The model under review builds one solid part; all positions refer to its coordinate system, in mm. A direction names the side the tool comes from. Round coordinates to 2 decimals unless told otherwise and drop trailing zeros. Write each loop counter-clockwise with the first axis right and the second up, starting at its lowest first coordinate (ties: lowest second). Pieces come first, ordered by that corner, then holes. Notation, with made-up numbers: M 80,59 L 117,59 A9 cw 117,68 Z; hole C -22,48.25 d6. An arc over 180 degrees is marked long. One line per item, written item: value. Start each with the question number.
1) Mouldability with a two-part tool opening along X and no side actions: class faces 1 (the face through (-128.15, 0, 37)), 2 (the face through (-142.35, -6.72, 22.98)), 3 (the face through (-146.05, 0, 61)) as +X half, -X half, draft (parallel to the pull), parting line (faces both ways), or undercut.
2) For P1, Ø13, axis at y = 0, z = 31.75, coming from the -X side; P2, Ø4, axis at x = -2, y = -10, coming from the +Z side; P3, Ø4, axis at x = 110.5, y = -12, coming from the -Z side, all flat-tipped, find the tip position at first contact; note any pin that passes through.
3) Take a section at D-D, the plane y = 0. State how many separate pieces and enclosed holes the cut face has, and give its area (3 significant figures).
4) Tool access review of faces 4 (the face through (-102, 0, 0)), 5 (the face through (-88, 0, 19.05)), 6 (the face through (-37.5, 0, -5)), 7 (the face through (101, 0, 0)), 8 (the face through (-133.42, 1.22, 35.61)): name each direction out of +Z, -Z, +X, -X, +Y, -Y from which nothing blocks a thin tool from reaching the whole face with its end or side.
5) Take a section at A-A, the plane x = -44.5. Write out the cut boundary in (y, z) (3 decimals), and give its area (3 significant figures).
6) Take a section at C-C, the plane z = 31.75. Write out the cut boundary in (x, y) (3 decimals), and give its area (3 significant figures).
7) Wall thickness on probe 1 along X at (y, z) = (11, 111.5); probe 2 along X at (y, z) = (-7, 38); probe 3 along X at (y, z) = (4, -11): over which ranges is each line inside the solid? List them lowest first.
8) Take a section at B-B, the plane z = 82. Write out the cut boundary in (x, y) (3 decimals).
from build123d import *

# Parameters (mm, degrees)
SKETCH1_R           = 8.05
SKETCH1_R_2         = 7
SKETCH1_R_3         = 1.25
BOSS_EXTRUDE1_DEPTH = 15.875
SKETCH2_R           = 11.05
CUT_EXTRUDE1_DEPTH  = 7.5
CUT_EXTRUDE3_START  = -7.5
SKETCH3_R           = 11.05
CUT_EXTRUDE3_DEPTH  = 7.5
SKETCH4_R           = 4.05
CUT_EXTRUDE4_DEPTH  = 10.4
SKETCH5_W           = 4
SKETCH5_H           = 27.75
CUT_EXTRUDE5_DEPTH  = 191.102710725


with BuildPart() as part:
    # Sketch1 → Boss-Extrude1 (new, symmetric)
    with BuildSketch(Plane(origin=(0, 0, 0), x_dir=(1, 0, 0), z_dir=(0, 1, 0))):
        with BuildLine():
            Line((-146.05, 0), (-56.5, 0))
            ThreePointArc((-56.5, 0), (-44.5, 12), (-32.5, 0))
            Line((-32.5, 0), (-15.05, 0))
            ThreePointArc((-15.05, 0), (0, 15.05), (15.05, 0))
            Line((15.05, 0), (32.5, 0))
            ThreePointArc((32.5, 0), (44.5, 12), (56.5, 0))
            Line((56.5, 0), (146.05, 0))
            Line((146.05, 0), (146.05, -120.65))
            Line((146.05, -120.65), (133.35, -120.65))
            Line((133.35, -120.65), (133.35, -44.45))
            Line((133.35, -44.45), (-57.15, -44.45))
            Line((-57.15, -44.45), (-57.15, -19.05))
            Line((-57.15, -19.05), (-120.65, -19.05))
            Line((-120.65, -19.05), (-120.65, -120.65))
            Line((-120.65, -120.65), (-146.05, -120.65))
            Line((-146.05, -120.65), (-146.05, 0))
        make_face()
        with Locations(Location((0, 0, 0), (0, 0, 270))):
            Circle(SKETCH1_R, mode=Mode.SUBTRACT)
        with Locations(Location((-44.5, 0, 0), (0, 0, 270))):
            Circle(SKETCH1_R_2, mode=Mode.SUBTRACT)
        with Locations(Location((44.5, 0, 0), (0, 0, 270))):
            Circle(SKETCH1_R_2, mode=Mode.SUBTRACT)
        with Locations(Location((0, 11.25, 0), (0, 0, 270))):
            Circle(SKETCH1_R_3, mode=Mode.SUBTRACT)
        with Locations(Location((9.742785793, -5.625, 0), (0, 0, 270))):
            Circle(SKETCH1_R_3, mode=Mode.SUBTRACT)
        with Locations(Location((-9.742785793, -5.625, 0), (0, 0, 270))):
            Circle(SKETCH1_R_3, mode=Mode.SUBTRACT)
    extrude(amount=BOSS_EXTRUDE1_DEPTH, both=True)

    # Sketch2 → Cut-Extrude1 (cut)
    with BuildSketch(Plane.ZY.offset(146.05)):
        with Locations((31.75, 0)):
            Circle(SKETCH2_R)
    extrude(amount=-CUT_EXTRUDE1_DEPTH, mode=Mode.SUBTRACT)

    # Sketch3 → Cut-Extrude3 (cut)
    with BuildSketch(Plane(origin=(-120.65, 0, 0), x_dir=(0, 0, -1), z_dir=(1, 0, 0)).offset(CUT_EXTRUDE3_START)):
        with Locations(Location((-31.75, 0, 0), (0, 0, 180))):
            Circle(SKETCH3_R)
    extrude(amount=CUT_EXTRUDE3_DEPTH, mode=Mode.SUBTRACT)

    # Sketch4 → Cut-Extrude4 (cut)
    with BuildSketch(Plane.ZY.offset(138.55)):
        with Locations((31.75, 0)):
            Circle(SKETCH4_R)
    extrude(amount=-CUT_EXTRUDE4_DEPTH, mode=Mode.SUBTRACT)

    # Sketch5 → Cut-Extrude5 (cut, through all)
    with BuildSketch(Plane(origin=(0, 0, 0), x_dir=(-1, 0, 0), z_dir=(0, 0, -1))):
        with Locations((-49.5, 0)):
            Rectangle(SKETCH5_W, SKETCH5_H)
        with Locations((-39.5, 0)):
            Rectangle(SKETCH5_W, SKETCH5_H)
        with Locations((49.5, 0)):
            Rectangle(SKETCH5_W, SKETCH5_H)
        with Locations((39.5, 0)):
            Rectangle(SKETCH5_W, SKETCH5_H)
    extrude(amount=CUT_EXTRUDE5_DEPTH, mode=Mode.SUBTRACT)


solid = part.part
Checked values:
1. face 1: undercut
1. face 2: draft
1. face 3: -X half
2. P1: stops at x = -138.55
2. P2: stops at z = 44.45
2. P3: stops at z = 0
3. separate pieces: 4
3. enclosed holes: 4
3. area: 14,000 mm2
4. face 4: -Z, -X, +Y, -Y
4. face 5: +Z, +Y, -Y
4. face 6: -Z
4. face 7: -Z, +X, +Y, -Y
4. face 8: -X
5. outline: M -15.875,-12 L 15.875,-12 L 15.875,-7 L -15.875,-7 Z; M -15.875,7 L 15.875,7 L 15.875,44.45 L -15.875,44.45 Z
5. area: 1,350 mm2
6. outline: M -146.05,-15.875 L -120.65,-15.875 L -120.65,-11.05 L -128.15,-11.05 L -128.15,-4.05 L -138.55,-4.05 L -138.55,-11.05 L -146.05,-11.05 Z; M -146.05,11.05 L -138.55,11.05 L -138.55,4.05 L -128.15,4.05 L -128.15,11.05 L -120.65,11.05 L -120.65,15.875 L -146.05,15.875 Z; M -57.15,-15.875 L 146.05,-15.875 L 146.05,15.875 L -57.15,15.875 Z
6. area: 6,840 mm2
7. probe 1: x = -146.05 to -120.65, 133.35 to 146.05
7. probe 2: x = -138.55 to -128.15, -57.15 to 146.05
7. probe 3: x = -47.5 to -41.5, -10.27 to -1.22, 1.22 to 10.27, 41.5 to 47.5
8. outline: M -146.05,-15.875 L -120.65,-15.875 L -120.65,15.875 L -146.05,15.875 Z; M 133.35,-15.875 L 146.05,-15.875 L 146.05,15.875 L 133.35,15.875 Z
